```python
from build123d import *

# Parameters (mm, degrees)
F0_W      = 12
F0_H      = 238
F0_H_2    = 12
F0_W_2    = 166
F0_H_3    = 272
F1_DEPTH  = 224
F2_R      = 24
F3_R      = 36
F5_DEPTH  = 12
F7_DEPTH  = 12
F8_R      = 63
F9_DEPTH  = 190
F10_R     = 11
F11_DEPTH = 25


with BuildPart() as f1:
    # F0 (on Front) → F1 (new body)
    with BuildSketch(Plane.XZ):
        with Locations((-29.668833, 69.198049)):
            Rectangle(F0_W, F0_H)
        with Locations((-29.668833, -55.801951)):
            Rectangle(F0_W, F0_H_2)
        with Locations((59.331167, -55.801951)):
            Rectangle(F0_W_2, F0_H_2)
        with Locations((148.331167, 86.198049)):
            Rectangle(F0_W, F0_H_3)
        with Locations((148.331167, -55.801951)):
            Rectangle(F0_W, F0_H_2)
    extrude(amount=F1_DEPTH)

    # F2
    f2_edges = [f1.edges().sort_by_distance(p)[0] for p in [
        (-23.668833, -112, -49.801951),
        (142.331167, -112, -49.801951),
    ]]
    fillet(f2_edges, radius=F2_R)

    # F3
    f3_edges = [f1.edges().sort_by_distance(p)[0] for p in [
        (154.331167, -112, -61.801951),
        (-35.668833, -112, -61.801951),
    ]]
    fillet(f3_edges, radius=F3_R)

    # F4 (on face) → F5 (cut)
    with BuildSketch(Plane(origin=(-35.668833, 0, 0), x_dir=(0, -1, 0), z_dir=(-1, 0, 0))):
        Polygon((0, 114.333307), (40, 188.198049), (0, 188.198049), align=None)
        Polygon((224, 188.198049), (184, 188.198049), (224, 114.333307), align=None)
    extrude(amount=-F5_DEPTH, mode=Mode.SUBTRACT)

    # F6 (on face) → F7 (cut)
    with BuildSketch(Plane.YZ.offset(154.331167)):
        Polygon((-224, 222.198049), (-224, 157.576071), (-184, 222.198049), align=None)
        Polygon((0, 222.198049), (-40, 222.198049), (0, 157.576071), align=None)
    extrude(amount=-F7_DEPTH, mode=Mode.SUBTRACT)

    # F8 (on face) → F9 (cut)
    with BuildSketch(Plane(origin=(-35.668833, 0, 0), x_dir=(0, -1, 0), z_dir=(-1, 0, 0))):
        with Locations((112, 113.482498)):
            Circle(F8_R)
    extrude(amount=-F9_DEPTH, mode=Mode.SUBTRACT)

    # F10 (on face) → F11 (cut)
    with BuildSketch(Plane.YZ.offset(154.331167)):
        with Locations((-166, 200.198049)):
            Circle(F10_R)
        with Locations((-58, 200.198049)):
            Circle(F10_R)
        with Locations((-34, 30.198049)):
            Circle(F10_R)
        with Locations((-190, 30.198049)):
            Circle(F10_R)
    extrude(amount=-F11_DEPTH, mode=Mode.SUBTRACT)


solid = f1.part
```
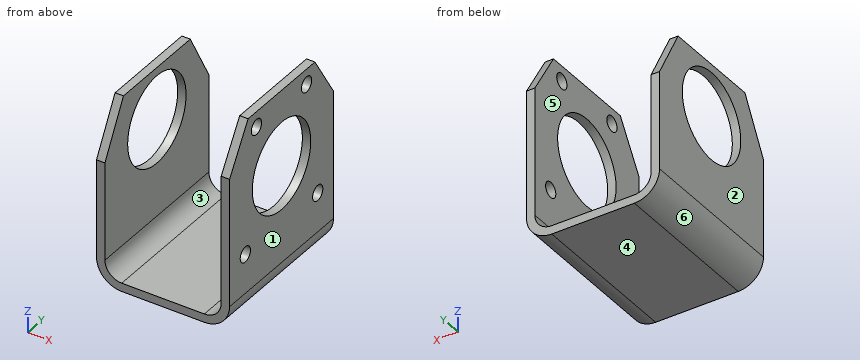
Can you work these out from the model? Positions are in its coordinate system, mm. Face numbers are marked on the shaded views. A direction names the side the tool comes from. Give positions to 0.01 mm unless a question says otherwise; leave off trailing zeros. Loops run counter-clockwise (first coordinate to the right, second up) from the corner with the lowest first, then second, coordinate; pieces in that order, holes last. Notation, with made-up numbers: M 46.5,-12.5 L 62.5,-12.5 A26 cw 62.5,19.5 Z; hole C 59,24 d4. An arc over 180 degrees is marked long. One line per item, written item: value.
(1) Suppose I cut it at A-A on z = 4.5. List the corners of the cut face in (x, y) for me, plus the area to 3 significant figures.
Returned:
outline: M -35.67,-224 L -23.67,-224 L -23.67,0 L -35.67,0 Z; M 142.33,-224 L 154.33,-224 L 154.33,0 L 142.33,0 Z
area: 5,380 mm^2
(2) Suppose I cut it at C-C on y = -168. List the corners of the cut face in (x, z) for me.
Returned:
outline: M -35.67,-25.8 A36 ccw 0.33,-61.8 L 118.33,-61.8 A36 ccw 154.33,-25.8 L 154.33,84.62 L 142.33,84.62 L 142.33,-25.8 A24 cw 118.33,-49.8 L 0.33,-49.8 A24 cw -23.67,-25.8 L -23.67,84.62 L -35.67,84.62 Z; M -35.67,142.34 L -23.67,142.34 L -23.67,188.2 L -35.67,188.2 Z; M 142.33,142.34 L 154.33,142.34 L 154.33,189.38 L 142.33,189.38 Z; M 142.33,211.01 L 154.33,211.01 L 154.33,222.2 L 142.33,222.2 Z
(3) Which directions (+Z, -Z, +X, -X, +Y, -Y) give clear straight access to the entire face, cutting with the end or side of a thin tool? Please do the marked faces 5 and 6.
Returned:
face 5: +Z, +Y, -Y
face 6: -Z, -X, +Y, -Y
(4) Will these pins go through, and if not, where does the flat tip stop? pin 1 (5 mm diameter, centred on x = -5.5, y = -35, fed in from -Z); pin 2 (6 mm diameter, centred on x = -31, y = -87, fed in from +Z); pin 3 (13 mm diameter, centred on y = -58, z = 200.2, fed in from +X).
Returned:
pin 1: z = -61.65
pin 2: z = 188.2
pin 3: through
(5) I need wall thicknesses on line 1 (X direction, y = -172, z = 56); line 2 (Z direction, x = 148.75, y = -166); line 3 (Z direction, x = 22.5, y = -106). Which ranges of each line are inside material? Lowest first, please.
Returned:
line 1: -35.67 to -23.67, 142.33 to 154.33
line 2: -45.06 to 81.03, 145.93 to 189.2, 211.2 to 222.2
line 3: -61.8 to -49.8
(6) Suppose I cut it at B-B on y = -112. List the corners of the cut face in (x, z) for me.
Returned:
outline: M -35.67,-25.8 A36 ccw 0.33,-61.8 L 118.33,-61.8 A36 ccw 154.33,-25.8 L 154.33,50.48 L 142.33,50.48 L 142.33,-25.8 A24 cw 118.33,-49.8 L 0.33,-49.8 A24 cw -23.67,-25.8 L -23.67,50.48 L -35.67,50.48 Z; M -35.67,176.48 L -23.67,176.48 L -23.67,188.2 L -35.67,188.2 Z; M 142.33,176.48 L 154.33,176.48 L 154.33,222.2 L 142.33,222.2 Z
(7) We'd pull the mould along X, two halves only. Please class the marked faces 1, 2, 3 and 4: released by +X, released by -X, zero draft, split by the parting line, or undercut.
Returned:
face 1: released by +X
face 2: released by -X
face 3: undercut
face 4: zero draft
(8) Suppose I cut it at D-D on y = -34. List the corners of the cut face in (x, z) for me.
Returned:
outline: M -35.67,-25.8 A36 ccw 0.33,-61.8 L 118.33,-61.8 A36 ccw 154.33,-25.8 L 154.33,19.2 L 142.33,19.2 L 142.33,-25.8 A24 cw 118.33,-49.8 L 0.33,-49.8 A24 cw -23.67,-25.8 L -23.67,177.12 L -35.67,177.12 Z; M 142.33,41.2 L 154.33,41.2 L 154.33,212.5 L 142.33,212.5 Z
